Geometry: final body of the model. Coordinates: model frame, mm. Face numbers are marked on the shaded views. Coordinates: 2 decimals unless noted, no trailing zeros. Write each loop counter-clockwise with the first axis right and the second up, starting at its lowest first coordinate (ties: lowest second). Pieces come first, ordered by that corner, then holes. Notation, with made-up numbers: M -26.5,64 L -8.5,64 A26 ccw -8.5,101 Z; hole C 64,5 d10. An arc over 180 degrees is marked long. Write item = value, one per line. Start each with the question number.
Item 1: Section A-A on x = 0. Output: boundary loops of the cut face in (y, z), plus the area to 3 significant figures.
Item 2: First-contact query: pin 1 Ø2 at (y, z) = (333.5, -5.5) entering from +X; pin 2 Ø3 at (x, y) = (-13.5, 197) entering from -Z; pin 3 Ø18 at (x, z) = (0, 0) entering from +Y; pin 4 Ø3 at (y, z) = (278, -23.5) entering from -X. Flat tips, straight axial feed; report the tip coordinate or a pass-through.
Item 3: Section B-B on z = 0. Output: boundary loops of the cut face in (x, y), plus the area to 3 significant figures.
Item 4: Section C-C on y = 69. Output: boundary loops of the cut face in (x, z), plus the area to 3 significant figures.
Item 5: Ray query, L1, parallel to X at y = 255, z = 0; L2, parallel to Y at x = -36, z = -22.5; L3, parallel to Z at x = 18, y = 36.5. Return the intervals inside material, ascending. Write a range as [from, to].
Item 6: Pull-direction query (X, two-part tool) for the marked faces 1, 2 and 3; classes: +X half, -X half, draft (parallel to the pull), parting line (faces both ways), or undercut.
from build123d import *

# Parameters (mm, degrees)
SKETCH1_R           = 42.5
BOSS_EXTRUDE1_DEPTH = 449.673299
SKETCH2_R           = 14.894380749
CUT_EXTRUDE1_DEPTH  = 454.672322093
CHAMFER1_SIZE       = 0.466639


with BuildPart() as part:
    # Sketch1 → Boss-Extrude1 (new body)
    with BuildSketch(Plane(origin=(0, 0, 0), x_dir=(1, 0, 0), z_dir=(0, 1, 0))):
        with Locations(Location((0, 0, 0), (0, 0, 270))):
            Circle(SKETCH1_R)
    extrude(amount=BOSS_EXTRUDE1_DEPTH)

    # Sketch2 → Cut-Extrude1 (cut, through all)
    with BuildSketch(Plane(origin=(0, 0, 0), x_dir=(1, 0, 0), z_dir=(0, 1, 0))):
        with Locations(Location((0, 0, 0), (0, 0, 270))):
            Circle(SKETCH2_R)
    extrude(amount=CUT_EXTRUDE1_DEPTH, mode=Mode.SUBTRACT)

    # Chamfer1
    chamfer1_edges = [part.edges().sort_by_distance(p)[0] for p in [
        (0, 0, -42.5),
        (0, 449.673299, -42.5),
    ]]
    chamfer(chamfer1_edges, length=CHAMFER1_SIZE)


solid = part.part
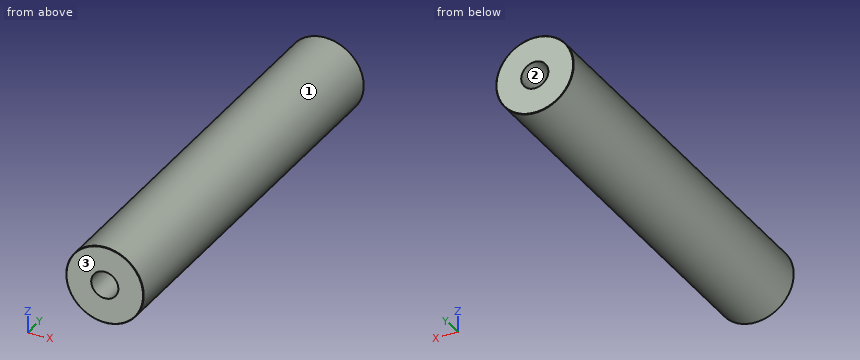
Responses:
q1.outline = M 0,-42.03 L 0.47,-42.5 L 449.21,-42.5 L 449.67,-42.03 L 449.67,-14.89 L 0,-14.89 Z; M 0,14.89 L 449.67,14.89 L 449.67,42.03 L 449.21,42.5 L 0.47,42.5 L 0,42.03 Z
q1.area = 24,800 mm²
q2.pin_1 = 42.26
q2.pin_2 = -40.77
q2.pin_3 = through
q2.pin_4 = -36.36
q3.outline = M -42.5,0.47 L -42.03,0 L -14.89,0 L -14.89,449.67 L -42.03,449.67 L -42.5,449.21 Z; M 14.89,0 L 42.03,0 L 42.5,0.47 L 42.5,449.21 L 42.03,449.67 L 14.89,449.67 Z
q3.area = 24,800 mm²
q4.outline = C 0,0 d85; hole C 0,0 d29.79
q4.area = 4,980 mm²
q5.L1 = [-42.5, -14.89], [14.89, 42.5]
q5.L2 = [0.42, 449.25]
q5.L3 = [-38.5, 38.5]
q6.face_1 = parting line
q6.face_2 = undercut
q6.face_3 = draft
